from build123d import *

# Parameters (mm, degrees)
THICKNESS_T = 1


with BuildPart() as part:
    # Sketch → Revolution (revolve)
    with BuildSketch(Plane.YZ):
        Polygon((0, 54.5), (2.5, 54.5), (2.5, 14.5), (5, 12), (5, 0), (0, 0), align=None)
    revolve(axis=Axis((0, 0, 0), (0, 0, 1)))

    # Thickness
    thickness_openings = [part.faces().sort_by_distance(p)[0] for p in [
        (0, 0, 54.5),
        (0, 0, 0),
    ]]
    offset(amount=THICKNESS_T, openings=thickness_openings)


solid = part.part
Input: part model. Units: mm. Frame: model coordinates. Coordinates: 2 decimals unless noted, no trailing zeros. Loops run counter-clockwise (first coordinate to the right, second up) from the corner with the lowest first, then second, coordinate; pieces in that order, holes last. Notation, with made-up numbers: (60, 19.5) -> (116, 19.5) arc R24 ccw to (116, 36.5) -> close; hole circle Ø7 at (73.25, -4.5). An arc over 180 degrees is marked (long way). Write each question's results on one line, items separated by ' | '. Start each with the question number.
Q1. Section C-C, the plane z = 44.5. Return the cut outline in (x, y), plus the area to 3 significant figures.
Q2. Pull-direction query (Y, two-part tool) for faces 1 (the flat face through (-4, -4, 0)), 2 (the cylindrical face through (1.341, 3.233, 34.43)), 3 (the cylindrical face through (4.88, -1.08, 5.92)); classes: released by +Y, released by -Y, zero draft, split by the parting line, or undercut.
Q3. Section A-A, the plane x = 0. Return the cut outline in (y, z).
Q4. Ray query, line 1 (Y direction, x = 0, z = 2.5); line 2 (X direction, y = 0, z = 36). Return the intervals inside material, ascending. Write a range as from..to.
Q5. Pin query (flat end, axial travel): pin 1 (1.5 mm diameter, centred on x = 1.5, z = 42.5, fed in from +Y); pin 2 (2 mm diameter, centred on x = 3, z = 40, fed in from +Y); pin 3 (1.5 mm diameter, centred on x = 2.5, y = 1.5, fed in from -Z); pin 4 (6 mm diameter, centred on x = 0.5, y = 3, fed in from -Z). Return the tip coordinate at first contact, or that it passes through.
Found:
1) outline: circle Ø7 at (0, 0); hole circle Ø5 at (0, 0) | area: 18.8 mm2
2) face 1: zero draft | face 2: split by the parting line | face 3: undercut
3) outline: (-6, 0) -> (-5, 0) -> (-5, 12) -> (-2.5, 14.5) -> (-2.5, 54.5) -> (-3.5, 54.5) -> (-3.5, 14.91) -> (-5.71, 12.71) arc R1 ccw to (-6, 12) -> close; (2.5, 14.5) -> (5, 12) -> (5, 0) -> (6, 0) -> (6, 12) arc R1 ccw to (5.71, 12.71) -> (3.5, 14.91) -> (3.5, 54.5) -> (2.5, 54.5) -> close
4) line 1: -6..-5, 5..6 | line 2: -3.5..-2.5, 2.5..3.5
5) pin 1: y = 3.42 | pin 2: y = 2.87 | pin 3: z = 13.33 | pin 4: z = 0
